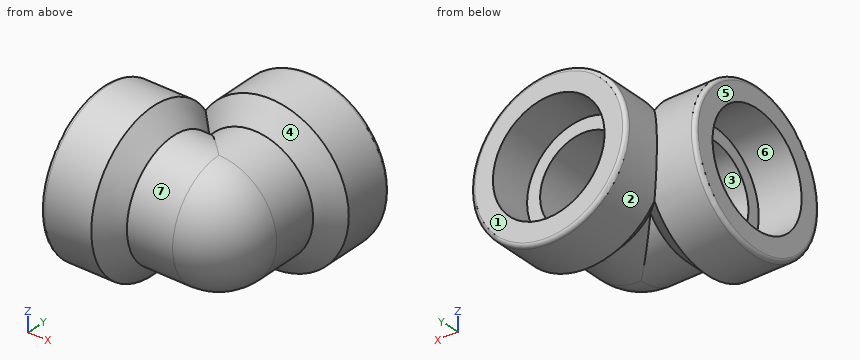
from build123d import *

# Parameters (mm, degrees)
CIRPATTERN2_COUNT  = 2
CIRPATTERN2_ANGLE  = 90
SKETCH4_R          = 12.954
CUT_EXTRUDE1_DEPTH = 55.857091
SKETCH5_R          = 12.954
CUT_EXTRUDE2_DEPTH = 55.857091
REVOLVE2_ANGLE     = 90


with BuildPart() as part:
    # Sketch2 → Revolve1 (revolve)
    with BuildSketch(Plane.XY, mode=Mode.PRIVATE) as revolve1_sk:
        with BuildLine():
            Line((-35.052, -16.891), (-22.098, -16.891))
            Line((-22.098, -16.891), (-22.098, -12.954))
            Line((-22.098, -12.954), (0, -12.954))
            Line((0, -12.954), (0, -17.5006))
            Line((0, -17.5006), (-13.8303, -17.5006))
            Line((-13.8303, -17.5006), (-19.8247, -23.495))
            Line((-19.8247, -23.495), (-33.91535, -23.495))
            ThreePointArc((-33.91535, -23.495), (-34.719082923, -23.162082923), (-35.052, -22.35835))
            Line((-35.052, -22.35835), (-35.052, -16.891))
        make_face()
    revolve(revolve1_sk.sketch.rotate(Axis((0, 0, 0), (-1, 0, 0)), 180), axis=Axis((0, 0, 0), (-1, 0, 0)))


with BuildPart() as cirpattern2_1:
    # CirPattern2: pattern copy
    add(part.part.rotate(Axis((0, 0, -23.495), (0, 0, -1)), 1 * CIRPATTERN2_ANGLE / (CIRPATTERN2_COUNT - 1)))

    # Sketch4 → Cut-Extrude1 (cut, through all)
    with BuildSketch(Plane(origin=(0, 0, 0), x_dir=(0, 0, -1), z_dir=(1, 0, 0))):
        with Locations(Location((0, 0, 0), (0, 0, 90))):
            Circle(SKETCH4_R)
    extrude(amount=-CUT_EXTRUDE1_DEPTH, mode=Mode.SUBTRACT)


with BuildPart() as part_1:
    add(part.part)

    # Sketch5 → Cut-Extrude2 (cut, through all)
    with BuildSketch(Plane.XZ):
        Circle(SKETCH5_R)
    extrude(amount=-CUT_EXTRUDE2_DEPTH, mode=Mode.SUBTRACT)

    # Combine1: union CirPattern2_1
    add(cirpattern2_1.part)

    # Sketch6 → Revolve2 (revolve)
    with BuildSketch(Plane(origin=(0, 0, 0), x_dir=(0, 0, -1), z_dir=(1, 0, 0))):
        with BuildLine():
            Line((-17.5006, 0), (-12.954, 0))
            ThreePointArc((-12.954, 0), (0, -12.954), (12.954, 0))
            Line((12.954, 0), (17.5006, 0))
            ThreePointArc((17.5006, 0), (0, -17.5006), (-17.5006, 0))
        make_face()
    revolve(axis=Axis((0, 0, 12.954), (0, 0, 1)), revolution_arc=REVOLVE2_ANGLE)


solid = part_1.part
For this review, take the finished solid that the model builds, in its own axes (mm). Face numbers are marked on the shaded views. A direction names the side the tool comes from. Round coordinates to 2 decimals unless told otherwise and drop trailing zeros. Order: outer loops, then holes, each group sorted by start corner. A loop starts at its lowest first (then second) coordinate and runs counter-clockwise, first axis right, second up. Notation, with made-up numbers: M 89.5,65 L 131.5,65 A6 ccw 131.5,75 Z; hole C 33.5,2 d10. An arc over 180 degrees is marked long. Use a Markdown table: item, result. Add a question column.
Item 1: Mouldability with a two-part tool opening along Z and no side actions: class the marked faces 5, 6 and 7 as released by +Z, released by -Z, zero draft, split by the parting line, or undercut.
Item 2: Insertion check: pin 1 (15.5 mm diameter, centred on x = 0, z = 0, fed in from +Y); pin 2 (3 mm diameter, centred on x = 12.5, y = 16.5, fed in from -Z); pin 3 (3 mm diameter, centred on y = 12, z = 11.5, fed in from +X). Each pin has a flat end and moves straight along its axis. Give the tip position at first contact, or say it passes through.
Item 3: Add section B-B, the plane y = 30. Give the boundary of the cut face in (x, z) (3 decimals).
Item 4: To check wall thickness, follow line 1 along Z through (x, y) = (0, 25.75) (3 decimals); line 2 along Z through (x, y) = (-9, 0); line 3 along X through (y, z) = (9.5, -16). State the ranges of each line that lie inside material, in increasing order.
Item 5: Tool access review of the marked faces 1, 2, 3 and 4: name each direction out of +Z, -Z, +X, -X, +Y, -Y from which nothing blocks a thin tool from reaching the whole face with its end or side.
Geometry results:
| question | item | result |
|---|---|---|
| 1 | face 5 | zero draft |
| 1 | face 6 | undercut |
| 1 | face 7 | split by the parting line |
| 2 | pin 1 | stops at y = -10.38 |
| 2 | pin 2 | stops at z = -17.97 |
| 2 | pin 3 | stops at x = 14.36 |
| 3 | outline | C 0,0 d46.99; hole C 0,0 d33.782 |
| 4 | line 1 | z = -23.495 to -16.891, 16.891 to 23.495 |
| 4 | line 2 | z = -17.5 to -12.95, 12.95 to 17.5 |
| 4 | line 3 | x = -35.05 to -14.94, -7.09 to 7.09 |
| 5 | face 1 | +Z, -Z, +X, -X, +Y |
| 5 | face 2 | +Y |
| 5 | face 3 | -X |
| 5 | face 4 | none |
